Geometry check sheet. Reference: the model listing, model coordinates, mm. Coordinates: 2 decimals unless noted, no trailing zeros. Loops run counter-clockwise (first coordinate to the right, second up) from the corner with the lowest first, then second, coordinate; pieces in that order, holes last.
Autodesk Inventor part; units mm, degrees
ref_plane "YZ Plane" through (0, 0, 0) normal (1, 0, 0) x (0, 1, 0)
ref_plane "XZ Plane" through (0, 0, 0) normal (0, 1, 0) x (-1, 0, 0)
ref_plane "XY Plane" through (0, 0, 0) normal (0, 0, 1) x (1, 0, 0)
sketch "Sketch1" plane through (0, 0, 0) normal (0, 0, 1) x (1, 0, 0)
  line L0 (-2.3812, -2.3813) -> (2.3813, -2.3813)
  line L1 (2.3813, -2.3813) -> (2.3812, 2.3812)
  line L2 (2.3812, 2.3812) -> (-2.3813, 2.3812)
  line L3 (-2.3813, 2.3812) -> (-2.3812, -2.3813)
  line L4 (-2.3812, -2.3813) -> (2.3812, 2.3812) construction
  line L5 (2.3813, -2.3813) -> (-2.3813, 2.3812) construction
  point P0 (0, 0)
  dimension "d0" = 4.7625
  dimension "d1" = 4.7625
extrude "Extrusion1" add sketch "Sketch1" along normal blind 11.1125
sketch "Sketch2" plane through (-2.3813, 2.3812, 0) normal (0, 1, 0) x (1, 0, 0)
  line L0 (2.3813, 0) -> (2.3813, -11.1125) construction
  line L1 (4.7625, -11.1125) -> (0, -11.1125)
  circle A0 centre (2.3813, -5.5563) radius 1.4732
  circle A1 centre (2.3813, -11.9062) radius 1.4732
  circle A2 centre (2.3813, -18.2563) radius 1.4732
  circle A3 centre (2.3813, -24.6063) radius 1.4732
  circle A4 centre (2.3813, -29.3688) radius 1.4493 construction
  line L2 (4.7625, 0) -> (0, 0)
  dimension "d4" = 2.9464
  dimension "d7" = 6.35
  dimension "d12" = 4.7625
  dimension "d13" = 5.5563
extrude "Extrusion2" cut sketch "Sketch2" against normal through all contours A0 | A2 | A3
sketch "Sketch3" plane through (2.3813, -2.3813, 0) normal (1, 0, 0) x (0, 0, -1)
  line L0 (0, 2.3813) -> (-11.1125, 2.3813) construction
  line L1 (-11.1125, 0) -> (-11.1125, 4.7625)
  circle A0 centre (-8.7312, 2.3813) radius 1.4732
  circle A1 centre (-2.3812, 2.3813) radius 1.4732
  circle A2 centre (3.9688, 2.3813) radius 1.4732
  circle A3 centre (10.3188, 2.3813) radius 1.4732
  dimension "d16" = 2.9464
  dimension "d17" = 2.3813
  dimension "d20" = 6.35
extrude "Extrusion3" cut sketch "Sketch3" against normal through all
chamfer "Chamfer1" distance 0.1 angle 45 4 edges at (-2.3813, 2.3812, 5.5563) (2.3812, 2.3812, 5.5563) (2.3813, -2.3813, 5.5563) (-2.3812, -2.3813, 5.5563)
equation "\"d1\" = d0"
properties part number "Nut Strip" material "Aluminum 6061"
(1) Sectioned sample at D-D on x = -1.7. Record the cut outline in (y, z).
Findings:
outline: (-2.38, 0) - (2.38, 0) - (2.38, 11.11) - (-2.38, 11.11) - close; hole circle Ø2.95 at (0, 2.38); hole circle Ø2.95 at (0, 8.73)
(2) Gauge pin test, flat end, axial feed: pin 1 Ø2.5 at (x, z) = (0, 5.56) entering from -Y. Record the tip position at first contact, or that the pin passes through.
Findings:
pin 1: passes through
(3) Sectioned sample at B-B on y = -0.6. Record the cut outline in (x, z), and give its area (3 significant figures).
Findings:
outline: (-2.38, 0) - (2.38, 0) - (2.38, 1.04) - (-2.38, 1.04) - close; (-2.38, 3.73) - (2.38, 3.73) - (2.38, 7.39) - (-2.38, 7.39) - close; (-2.38, 10.08) - (2.38, 10.08) - (2.38, 11.11) - (-2.38, 11.11) - close; hole circle Ø2.95 at (0, 5.56)
area: 20.5 mm2
(4) Sectioned sample at A-A on x = 0. Record the cut outline in (y, z).
Findings:
outline: (-2.38, 0) - (2.38, 0) - (2.38, 4.08) - (-2.38, 4.08) - close; (-2.38, 7.03) - (2.38, 7.03) - (2.38, 11.11) - (-2.38, 11.11) - close; hole circle Ø2.95 at (0, 2.38); hole circle Ø2.95 at (0, 8.73)
(5) Scan lines: L1, parallel to Z at x = 0.65, y = 0; L2, parallel to Z at x = 1.7, y = -1.35; L3, parallel to Z at x = -0.95, y = -0.5. Record each from-to range of solid material in increasing order.
Findings:
L1: z = 0 to 0.91, 3.85 to 4.23, 6.88 to 7.26, 10.2 to 11.11
L2: z = 0 to 1.79, 2.97 to 8.14, 9.32 to 11.11
L3: z = 0 to 1, 3.77 to 4.43, 6.68 to 7.35, 10.12 to 11.11
(6) Sectioned sample at C-C on z = 4.5. Record the cut outline in (x, y), and give its area (3 significant figures).
Findings:
outline: (-2.38, -2.28) - (-2.28, -2.38) - (-1.03, -2.38) - (-1.03, 2.38) - (-2.28, 2.38) - (-2.38, 2.28) - close; (1.03, -2.38) - (2.28, -2.38) - (2.38, -2.28) - (2.38, 2.28) - (2.28, 2.38) - (1.03, 2.38) - close
area: 12.9 mm2
(7) Draft check along Z on faces 1 (the flat face through (2, 2.381, 5)), 2 (the cylindrical face through (0.033, 0.443, 7.326)), 3 (the flat face through (0, 0, 11.112)), 4 (the cylindrical face through (0.03, -0.9, 3.55)). Enter one of: +Z half, -Z half, draft (parallel to the pull), parting line (faces both ways), or undercut.
Findings:
face 1: draft
face 2: undercut
face 3: +Z half
face 4: undercut
